Here's how the part is built. I have some questions about the finished solid (model axes, mm). Face numbers are marked on the shaded views. A direction names the side the tool comes from. Coordinates: 2 decimals unless noted, no trailing zeros. Order: outer loops, then holes, each group sorted by start corner. A loop starts at its lowest first (then second) coordinate and runs counter-clockwise, first axis right, second up. Notation, with made-up numbers: (67.5, 24) - (73.5, 24) arc R24 cw to (73.5, 35) - close; hole circle Ø6 at (-4.75, -15). An arc over 180 degrees is marked (long way). Answer as CSV lines item,"result". Start each with the question number.
Q1. Suppose I cut it at D-D (x = 7.25). Please give me the cut outline in (y, z).
Q2. Suppose I cut it at A-A (x = 0). Count the separate pieces of the cut face and the enclosed holes in it, then the cut area to 3 significant figures.
Q3. For pin 1 Ø3 at (y, z) = (13, 5) entering from +X; pin 2 Ø6 at (x, y) = (2, 12) entering from +Z; pin 3 Ø0.7 at (y, z) = (1, 14.5) entering from -X; pin 4 Ø1.1 at (y, z) = (13, 1.5) entering from +X, each with a flat end and sliding along its axis, tell me the tip position at first contact or that it passes through.
Q4. I need wall thicknesses on line 1 (X direction, y = 18, z = 4.5); line 2 (Y direction, x = -6.25, z = 12.75). Which ranges of each line are inside material? Lowest first, please.
Q5. Suppose I cut it at B-B (x = -4.5). Please give me the cut outline in (y, z), then the cut area to 3 significant figures.
Q6. Suppose I cut it at C-C (z = 21.75). Please give me the cut outline in (x, y).
Q7. Thinking about a two-plate mould opening in X: for the marked faces 1, 2 and 3, which applies, released by +X, released by -X, zero draft, split by the parting line, or undercut?
Q8. For the marked faces 4 and 5, which set-ups out of +Z, -Z, +X, -X, +Y, -Y let a thin tool reach every point of the face, with its end or its side?
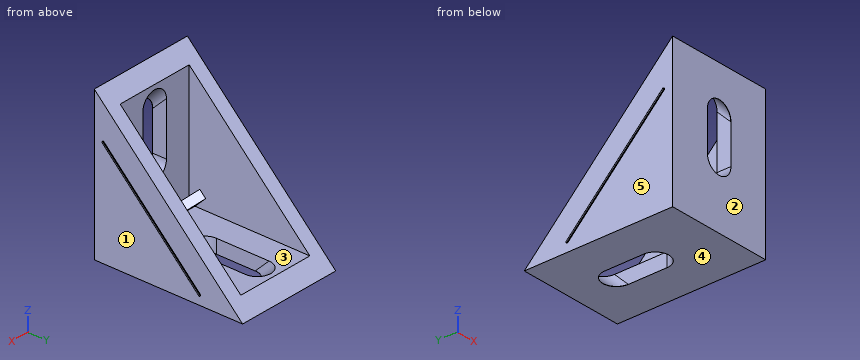
from build123d import *

# Parameters (mm, degrees)
BOSS_EXTRUDE1_DEPTH      = 8.5
BOSS_EXTRUDE1_DEPTH_BACK = 8.5
SHELL1_T                 = -2.2
BOSS_EXTRUDE2_DEPTH      = 0.66
CUT_EXTRUDE1_REACH       = 36.441
CUT_EXTRUDE2_REACH       = 36.441
EXTRUDE_THIN1_DEPTH      = 0.1
FILLET1_R                = 0.127
FILLET2_R                = 0.0508
FILLET1_OF_MIRROR1_R     = 0.127
FILLET2_OF_MIRROR1_R     = 0.0508


with BuildPart() as part:
    # Sketch4 → Boss-Extrude1 (new, two sides: drawn at the far end of the back side and taken through both)
    with BuildSketch(Plane(origin=(0, 0, 0), x_dir=(0, 0, -1), z_dir=(1, 0, 0)).offset(-BOSS_EXTRUDE1_DEPTH_BACK)):
        Polygon((0, 0), (-23.6, 0), (0, 23.6), align=None)
    extrude(amount=BOSS_EXTRUDE1_DEPTH + BOSS_EXTRUDE1_DEPTH_BACK)

    # Shell1
    shell1_openings = [part.faces().sort_by_distance(p)[0] for p in [
        (0, 11.8, 11.8),
    ]]
    offset(amount=SHELL1_T, openings=shell1_openings, kind=Kind.INTERSECTION)

    # Sketch5 → Boss-Extrude2 (add, symmetric)
    with BuildSketch(Plane(origin=(0, 0, 0), x_dir=(1, 0, 0), z_dir=(0, 0.7071067811865477, -0.7071067811865474))):
        Polygon((6.3, -3.111269837), (1.728, -3.111269837), (6.3, -6.159269837), align=None)
        Polygon((-1.728, -3.111269837), (-6.3, -6.159269837), (-6.3, -3.111269837), align=None)
    extrude(amount=BOSS_EXTRUDE2_DEPTH, both=True)

    # Sketch9 → Cut-Extrude1 (cut, up to next)
    with BuildSketch(Plane.XZ, mode=Mode.PRIVATE) as cut_extrude1_sk1:
        with BuildLine():
            Line((-2.15, 10.15), (-2.15, 16.35))
            ThreePointArc((-2.15, 16.35), (0, 18.5), (2.15, 16.35))
            Line((2.15, 16.35), (2.15, 10.15))
            ThreePointArc((2.15, 10.15), (0, 8), (-2.15, 10.15))
        make_face()
    cut_extrude1_tool1 = extrude(cut_extrude1_sk1.sketch, amount=-CUT_EXTRUDE1_REACH, mode=Mode.PRIVATE) & part.part
    add(cut_extrude1_tool1.solids().sort_by_distance((0, 0, 13.25))[0], mode=Mode.SUBTRACT)

    # Cut-Sweep2: sweep along a path in Sketch8
    with BuildLine(Plane(origin=(0, 0, 0), x_dir=(0, 0, -1), z_dir=(1, 0, 0))) as cut_sweep2_path:
        Line((-20.7, 2.2), (-18.5, 0))
    # Sketch10 → Cut-Sweep2 (sweep, cut)
    with BuildSketch(Plane(origin=(0, 2.2, 0), x_dir=(1, 0, 0), z_dir=(0, 1, 0))):
        with BuildLine():
            Line((-2.15, -18.519), (-2.15, -16.35))
            Line((-2.15, -16.35), (2.15, -16.35))
            Line((2.15, -16.35), (2.15, -18.519))
            ThreePointArc((2.15, -18.519), (0, -20.669), (-2.15, -18.519))
        make_face()
    sweep(path=cut_sweep2_path.line, mode=Mode.SUBTRACT)

    # Sketch11 → Cut-Extrude2 (cut, up to next)
    with BuildSketch(Plane(origin=(0, 0, 0), x_dir=(-1, 0, 0), z_dir=(0, 0, -1)), mode=Mode.PRIVATE) as cut_extrude2_sk1:
        with BuildLine():
            Line((-2.15, 16.35), (-2.15, 10.15))
            ThreePointArc((-2.15, 10.15), (0, 8), (2.15, 10.15))
            Line((2.15, 10.15), (2.15, 16.35))
            ThreePointArc((2.15, 16.35), (0, 18.5), (-2.15, 16.35))
        make_face()
    cut_extrude2_tool1 = extrude(cut_extrude2_sk1.sketch, amount=-CUT_EXTRUDE2_REACH, mode=Mode.PRIVATE) & part.part
    add(cut_extrude2_tool1.solids().sort_by_distance((0, 13.25, 0))[0], mode=Mode.SUBTRACT)

    # Cut-Sweep3: sweep along a path in Sketch13
    with BuildLine(Plane(origin=(0, 0, 0), x_dir=(0, 0, -1), z_dir=(1, 0, 0))) as cut_sweep3_path:
        Line((-2.2, 20.7), (0, 18.5))
    # Sketch12 → Cut-Sweep3 (sweep, cut)
    with BuildSketch(Plane.XY.offset(2.2)):
        with BuildLine():
            Line((-2.15, 18.519), (-2.15, 16.35))
            Line((-2.15, 16.35), (2.15, 16.35))
            Line((2.15, 16.35), (2.15, 18.519))
            ThreePointArc((2.15, 18.519), (0, 20.669), (-2.15, 18.519))
        make_face()
    sweep(path=cut_sweep3_path.line, mode=Mode.SUBTRACT)

    # Sketch14 → Extrude-Thin1 (add)
    with BuildSketch(Plane(origin=(8.5, 0, 0), x_dir=(0, 0, -1), z_dir=(1, 0, 0))):
        Polygon((-1.435511644, 16.99186083), (-16.99186083, 1.435511644), (-16.776334683, 1.219985497), (-1.219985497, 16.776334683), align=None)
    extrude_thin1 = extrude(amount=EXTRUDE_THIN1_DEPTH)

    # Fillet1
    fillet1_edges = [part.edges().sort_by_distance(p)[0] for p in [
        (8.55, 16.99186083, 1.435511644),
        (8.55, 1.435511644, 16.99186083),
        (8.55, 1.219985497, 16.776334683),
        (8.55, 16.776334683, 1.219985497),
    ]]
    fillet(fillet1_edges, radius=FILLET1_R)

    # Fillet2
    fillet2_edges = [part.edges().sort_by_distance(p)[0] for p in [
        (8.6, 9.213686237, 9.213686237),
        (8.6, 16.884097757, 1.327748571),
        (8.6, 1.327748571, 16.884097757),
        (8.6, 8.99816009, 8.99816009),
        (8.6, 1.435511644, 16.939255708),
        (8.6, 1.27259062, 16.776334683),
        (8.6, 16.776334683, 1.27259062),
        (8.6, 16.939255708, 1.435511644),
    ]]
    fillet(fillet2_edges, radius=FILLET2_R)

    # Mirror1: Extrude-Thin1 across plane
    add(extrude_thin1.mirror(Plane(origin=(0, 0, 0), x_dir=(0, 0, 1), z_dir=(1, 0, 0))))

    # Fillet1 of Mirror1
    fillet1_of_mirror1_edges = [part.edges().sort_by_distance(p)[0] for p in [
        (-8.55, 16.99186083, 1.435511644),
        (-8.55, 1.435511644, 16.99186083),
        (-8.55, 1.219985497, 16.776334683),
        (-8.55, 16.776334683, 1.219985497),
    ]]
    fillet(fillet1_of_mirror1_edges, radius=FILLET1_OF_MIRROR1_R)

    # Fillet2 of Mirror1
    fillet2_of_mirror1_edges = [part.edges().sort_by_distance(p)[0] for p in [
        (-8.6, 9.213686237, 9.213686237),
        (-8.6, 16.884097757, 1.327748571),
        (-8.6, 1.327748571, 16.884097757),
        (-8.6, 8.99816009, 8.99816009),
        (-8.6, 1.435511644, 16.939255708),
        (-8.6, 1.27259062, 16.776334683),
        (-8.6, 16.776334683, 1.27259062),
        (-8.6, 16.939255708, 1.435511644),
    ]]
    fillet(fillet2_of_mirror1_edges, radius=FILLET2_OF_MIRROR1_R)


solid = part.part
Here are the results:
1,outline,"(0, 0) - (23.6, 0) - (0, 23.6) - close"
2,separate pieces,"3"
2,enclosed holes,"0"
2,area,"43.3 mm²"
3,pin 1,"stops at x = 8.6"
3,pin 2,"stops at z = 2.2"
3,pin 3,"stops at x = -8.5"
3,pin 4,"stops at x = 8.5"
4,line 1,"x = -8.5 to -6.3, 6.3 to 8.5"
4,line 2,"y = 0 to 2.2"
5,outline,"(0, 0) - (23.6, 0) - (21.4, 2.2) - (3.13, 2.2) - (3.97, 3.04) - (3.04, 3.97) - (2.2, 3.13) - (2.2, 21.4) - (0, 23.6) - close"
5,area,"96.2 mm²"
6,outline,"(-8.5, 0) - (8.5, 0) - (8.5, 1.85) - (-8.5, 1.85) - close"
7,face 1,"released by +X"
7,face 2,"zero draft"
7,face 3,"undercut"
8,face 4,"-Z, +X, -X, +Y, -Y"
8,face 5,"-X"
